Read the model definition and answer for the solid it produces. Units are mm, in the model's axes. Face numbers are marked on the shaded views. Coordinates: 2 decimals unless noted, no trailing zeros. Write each loop counter-clockwise with the first axis right and the second up, starting at its lowest first coordinate (ties: lowest second). Pieces come first, ordered by that corner, then holes.
(1) Determine the mould class of the marked faces 1 and 2 for opening direction Z: pulls with the +Z half, pulls with the -Z half, needs draft (parallel to the pull), parting line crosses it, or undercut.
(2) The part is cut by section A-A, the plane y = -37.5. Determine the outline of the cut face in (x, z).
(3) Given pin 1 (3 mm diameter, centred on x = -10, y = -58, fed in from -Z); pin 2 (16.5 mm diameter, centred on x = 12.5, z = -7, fed in from -Y); pin 3 (8 mm diameter, centred on x = 7.5, y = -153.5, fed in from +Z), each flat-ended and moving along its own axis, determine where each tip first touches the part or whether it passes through.
(4) Straight lines are drawn through the part: line 1 along Z through (x, y) = (7, -165); line 2 along X through (y, z) = (-60, -22); line 3 along Z through (x, y) = (20, -88). For each, find the intervals that lie inside material, in ascending order.
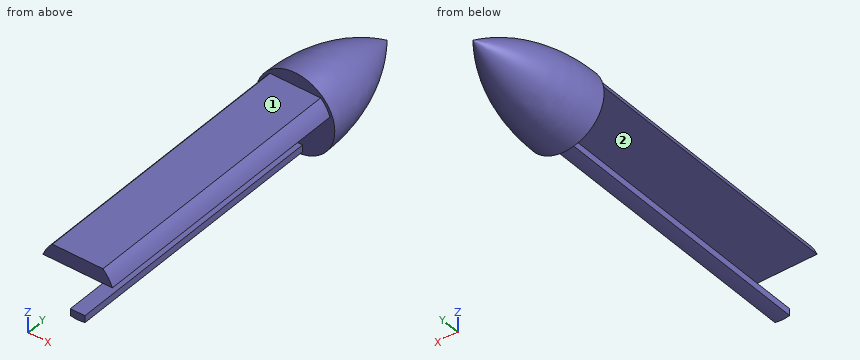
```python
from build123d import *

# Parameters (mm, degrees)
SKETCH3_R           = 25.2
BOSS_EXTRUDE1_DEPTH = 190
CUT_EXTRUDE1_START  = -190
CUT_EXTRUDE1_DEPTH  = 190


with BuildPart() as part:
    # Sketch2 → Revolve1 (revolve)
    with BuildSketch(Plane.XY):
        with BuildLine():
            Line((0, 0), (0, 80))
            add(Edge.make_bspline(
                [(0, 80), (26.841301525, 45.581737531), (27.1, 0)],
                knots=[0, 0, 0, 1, 1, 1], degree=2))
            Line((27.1, 0), (0, 0))
        make_face()
    revolve(axis=Axis((0, 0, 0), (0, 1, 0)))

    # Sketch3 → Boss-Extrude1 (add)
    with BuildSketch(Plane.XZ):
        with Locations(Location((0, 0, 0), (0, 0, 270))):
            Circle(SKETCH3_R)
    extrude(amount=BOSS_EXTRUDE1_DEPTH)

    # Sketch4 → Cut-Extrude1 (cut)
    with BuildSketch(Plane.XZ.offset(190).offset(CUT_EXTRUDE1_START)):
        with BuildLine():
            Line((-23.811289339, -8.25), (0, -8.25))
            Line((0, -8.25), (23.811289339, -8.25))
            ThreePointArc((23.811289339, -8.25), (24.850397294, -4.183031715), (25.2, 0))
            ThreePointArc((25.2, 0), (24.850397294, 4.183031715), (23.811289339, 8.25))
            Line((23.811289339, 8.25), (-23.811289339, 8.25))
            ThreePointArc((-23.811289339, 8.25), (-25.2, 0), (-23.811289339, -8.25))
        make_face()
        with BuildLine():
            Line((0, -20), (0, -8.25))
            Line((0, -8.25), (-23.811289339, -8.25))
            ThreePointArc((-23.811289339, -8.25), (-16.588095085, -18.97037431), (-5, -24.698987834))
            Line((-5, -24.698987834), (-5, -20))
            Line((-5, -20), (0, -20))
        make_face()
        with BuildLine():
            Line((23.811289339, -8.25), (0, -8.25))
            Line((0, -8.25), (0, -20))
            Line((0, -20), (5, -20))
            Line((5, -20), (5, -24.698987834))
            ThreePointArc((5, -24.698987834), (16.588095085, -18.97037431), (23.811289339, -8.25))
        make_face()
        with BuildLine():
            ThreePointArc((17.37749982, 18.25), (0, 25.2), (-17.37749982, 18.25))
            Line((-17.37749982, 18.25), (17.37749982, 18.25))
        make_face()
    extrude(amount=CUT_EXTRUDE1_DEPTH, mode=Mode.SUBTRACT)


solid = part.part
```
Computed:
1. face 1: pulls with the +Z half
1. face 2: undercut
2. outline: (-23.81, 8.25) - (23.81, 8.25) arc R25.2 ccw to (17.38, 18.25) - (-17.38, 18.25) arc R25.2 ccw to start; (-5, -24.7) arc R25.2 ccw to (5, -24.7) - (5, -20) - (-5, -20) - close
3. pin 1: stops at z = 8.25
3. pin 2: stops at y = 0
3. pin 3: stops at z = 18.25
4. line 1: z = 8.25 to 18.25
4. line 2: x = -5 to 5
4. line 3: z = 8.25 to 15.33
